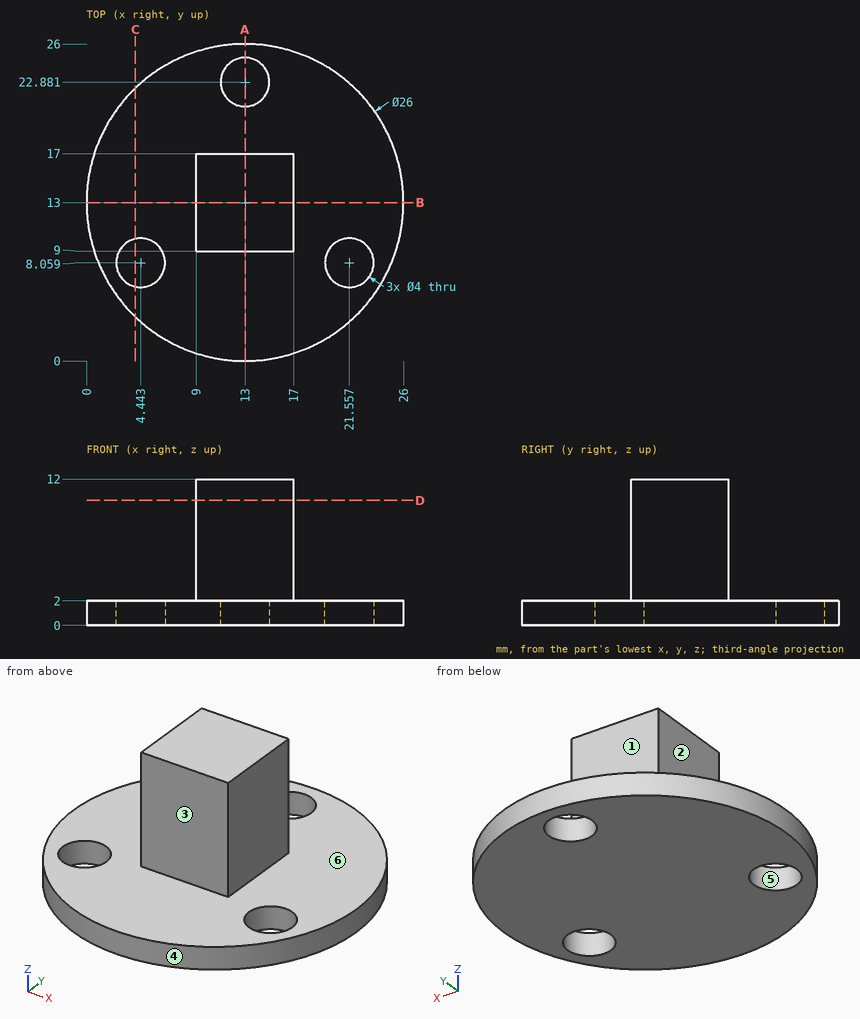
Could you check a few things on this drawing? It's one solid part, dimensions in mm from its lowest x, y, z. A direction names the side the tool comes from. Coordinates: 2 decimals unless noted, no trailing zeros. Write each loop counter-clockwise with the first axis right and the second up, starting at its lowest first coordinate (ties: lowest second). Pieces come first, ordered by that corner, then holes.
1) If we section it at D-D (z = 10.25): List the corners of the cut face in (x, y) for me, plus the area to 3 significant figures.
Filled in:
outline: (9, 9) - (17, 9) - (17, 17) - (9, 17) - close
area: 64.0 mm2
2) If we section it at B-B (y = 13): List the corners of the cut face in (x, z) for me, plus the area to 3 significant figures.
Filled in:
outline: (0, 0) - (26, 0) - (26, 2) - (17, 2) - (17, 12) - (9, 12) - (9, 2) - (0, 2) - close
area: 132 mm2
3) Thinking about a two-plate mould opening in Y: for the marked faces 4, 5 and 6, which applies, +Y half, -Y half, draft (parallel to the pull), parting line (faces both ways), or undercut?
Filled in:
face 4: parting line
face 5: undercut
face 6: draft
4) If I drill on line 1 (Y direction, x = 13, z = 0.9); line 2 (Y direction, x = 12.5, z = 3.25); line 3 (Z direction, x = 18, y = 3.5), over which ranges is the centre line in solid material (lowest first)?
Filled in:
line 1: y = 0 to 20.88, 24.88 to 26
line 2: y = 9 to 17
line 3: z = 0 to 2
5) If we section it at A-A (x = 13): List the corners of the cut face in (y, z) for me.
Filled in:
outline: (0, 0) - (20.88, 0) - (20.88, 2) - (17, 2) - (17, 12) - (9, 12) - (9, 2) - (0, 2) - close; (24.88, 0) - (26, 0) - (26, 2) - (24.88, 2) - close
6) Which directions (+Z, -Z, +X, -X, +Y, -Y) give clear straight access to the entire face, cutting with the end or side of a thin tool? Please do the marked faces 1, 2 and 3.
Filled in:
face 1: +Z, +X, -X, +Y
face 2: +Z, -X, +Y, -Y
face 3: +Z, +X, -X, -Y
7) I'm going to push flat-ended pins straight in: pin 1 (2.5 mm diameter, centred on x = 14.5, z = 8, fed in from +Y); pin 2 (4 mm diameter, centred on y = 11.5, z = 8.5, fed in from +X); pin 3 (6.5 mm diameter, centred on x = 4.44, y = 8.06, fed in from +Z). Where does each tip first touch, or does it pass through?
Filled in:
pin 1: stops at y = 17
pin 2: stops at x = 17
pin 3: stops at z = 2
8) If we section it at C-C (x = 4): List the corners of the cut face in (y, z) for me.
Filled in:
outline: (3.62, 0) - (6.11, 0) - (6.11, 2) - (3.62, 2) - close; (10.01, 0) - (22.38, 0) - (22.38, 2) - (10.01, 2) - close
